```python
from build123d import *

# Parameters (mm, degrees)
SKETCH_W     = 23
SKETCH_H     = 23
PAD_DEPTH    = 1.8
SKETCH001_W  = 20.6
SKETCH001_H  = 20.6
PAD001_DEPTH = 1.2
POCKET_DEPTH = 5


with BuildPart() as part:
    # Sketch → Pad (new body)
    with BuildSketch(Plane.XY):
        Rectangle(SKETCH_W, SKETCH_H)
    extrude(amount=PAD_DEPTH)

    # Sketch001 (on Face6 of Pad) → Pad001 (join)
    with BuildSketch(Plane.XY.offset(1.8)):
        Rectangle(SKETCH001_W, SKETCH001_H)
    extrude(amount=PAD001_DEPTH)

    # Sketch002 (on Face4 of Pad001) → Pocket (cut)
    with BuildSketch(Plane(origin=(0, 0, 0), x_dir=(1, 0, 0), z_dir=(0, 0, -1))):
        with BuildLine():
            ThreePointArc((2.5, -5), (0, -2.5), (-2.5, -5))
            Line((-2.5, -5), (-2.5, -13.46))
            ThreePointArc((-2.5, -13.46), (0, -15.96), (2.5, -13.46))
            Line((2.5, -13.46), (2.5, -5))
        make_face()
    extrude(amount=-POCKET_DEPTH, mode=Mode.SUBTRACT)


solid = part.part
```
Build history of the part. All positions in model axes, mm. A direction names the side the tool comes from. Coordinates: 2 decimals unless noted, no trailing zeros. Write each loop counter-clockwise with the first axis right and the second up, starting at its lowest first coordinate (ties: lowest second). Pieces come first, ordered by that corner, then holes.
1. Band-saw the part on D-D, the plane x = 0. Give the cut face in (y, z), and give its area (3 significant figures).
Answer block:
outline: (-11.5, 0) - (2.5, 0) - (2.5, 3) - (-10.3, 3) - (-10.3, 1.8) - (-11.5, 1.8) - close
area: 40.6 mm2
2. Drill centre lines: probe 1 along X at (y, z) = (7, 2.3); probe 2 along Y at (x, z) = (7, 2.75). Where is each one in solid material? Low to high.
Answer block:
probe 1: x = -10.3 to -2.5, 2.5 to 10.3
probe 2: y = -10.3 to 10.3
3. 3-axis set-ups, long thin cutter, end or side, ignore diameter. For faces 1 (the flat face through (10.3, 0, 2)), 2 (the flat face through (-10.3, 0, 2)), 3 (the flat face through (2.5, 8, 1)), 4 (the flat face through (6, 10.3, 2)): which of +Z, -Z, +X, -X, +Y, -Y reach the whole face in a straight line?
Answer block:
face 1: +Z, +X, +Y, -Y
face 2: +Z, -X, +Y, -Y
face 3: +Z, -Z, +Y
face 4: +Z, +X, -X, +Y
4. Band-saw the part on C-C, the plane x = 4.25. Give the cut face in (y, z), and give its area (3 significant figures).
Answer block:
outline: (-11.5, 0) - (11.5, 0) - (11.5, 1.8) - (10.3, 1.8) - (10.3, 3) - (-10.3, 3) - (-10.3, 1.8) - (-11.5, 1.8) - close
area: 66.1 mm2
5. Band-saw the part on B-B, the plane z = 0.65. Give the cut face in (x, y), and give its area (3 significant figures).
Answer block:
outline: (-11.5, -11.5) - (11.5, -11.5) - (11.5, 11.5) - (2.5, 11.5) - (2.5, 5) arc R2.5 cw to (-2.5, 5) - (-2.5, 11.5) - (-11.5, 11.5) - close
area: 487 mm2
6. Drop flat-ended pins along their axis: pin 1 (1.3 mm diameter, centred on x = 1, z = 2.5, fed in from -Y); pin 2 (1 mm diameter, centred on y = 0, z = 2.5, fed in from -X); pin 3 (1 mm diameter, centred on x = 1, z = 0.5, fed in from +Y). Give the stop position or say it passes through.
Answer block:
pin 1: stops at y = -10.3
pin 2: stops at x = -10.3
pin 3: stops at y = 3
7. Band-saw the part on A-A, the plane y = 6.75. Give the cut face in (x, z).
Answer block:
outline: (-11.5, 0) - (-2.5, 0) - (-2.5, 3) - (-10.3, 3) - (-10.3, 1.8) - (-11.5, 1.8) - close; (2.5, 0) - (11.5, 0) - (11.5, 1.8) - (10.3, 1.8) - (10.3, 3) - (2.5, 3) - close
8. Pull direction X, two halves, no side cores. Call faces 5 (the flat face through (-2.5, 8, 1)), 6 (the cylindrical face through (0.1, 2.5, 1.5)), 7 (the flat face through (0, -10.3, 2)), 8 (the flat face through (11.5, 0, 1)): released by +X, released by -X, zero draft, split by the parting line, or undercut.
Answer block:
face 5: undercut
face 6: undercut
face 7: zero draft
face 8: released by +X
